The drawing under review shows one solid part. Ordinate dimensions are in mm from its lowest x, y, z. A direction names the side the tool comes from. Coordinates: 2 decimals unless noted, no trailing zeros. Write each loop counter-clockwise with the first axis right and the second up, starting at its lowest first coordinate (ties: lowest second). Pieces come first, ordered by that corner, then holes. Notation, with made-up numbers: (82.25, -2.75) - (129.25, -2.75) arc R19 ccw to (129.25, 33.25) - close; hole circle Ø10 at (5.25, -5). An arc over 180 degrees is marked (long way). Put each result on its own line as item: value. Start each with the question number.
Item 1: Machinability: for the marked faces 1 and 2, which of the approach directions +Z, -Z, +X, -X, +Y, -Y give a long, thin tool a straight path to every point of the face, cutting with its end or side? Answer none if there is none.
Item 2: Consider section B-B on z = 7.5. Give the boundary of the cut face in (x, y), then the cut area to 3 significant figures.
Item 3: Consider section A-A on x = 5.25. Give the boundary of the cut face in (y, z), then the cut area to 3 significant figures.
Item 4: To check wall thickness, follow L1, parallel to Y at x = 19, z = 1.5; L2, parallel to X at y = 37.5, z = 3.75; L3, parallel to Y at x = 11.25, z = 8. State the ranges of each line that lie inside material, in increasing order. Write a range as [from, to].
Item 5: Mouldability with a two-part tool opening along X and no side actions: class the marked faces 3, 4 and 5 as pulls with the +X half, pulls with the -X half, needs draft (parallel to the pull), parting line crosses it, or undercut.
Item 6: Consider section C-C on y = 33.5. Give the boundary of the cut face in (x, z).
Item 7: For pin 1 (10 mm diameter, centred on x = 10, y = 11, fed in from +Z), flat-tipped, find the tip position at first contact; note if it passes through.
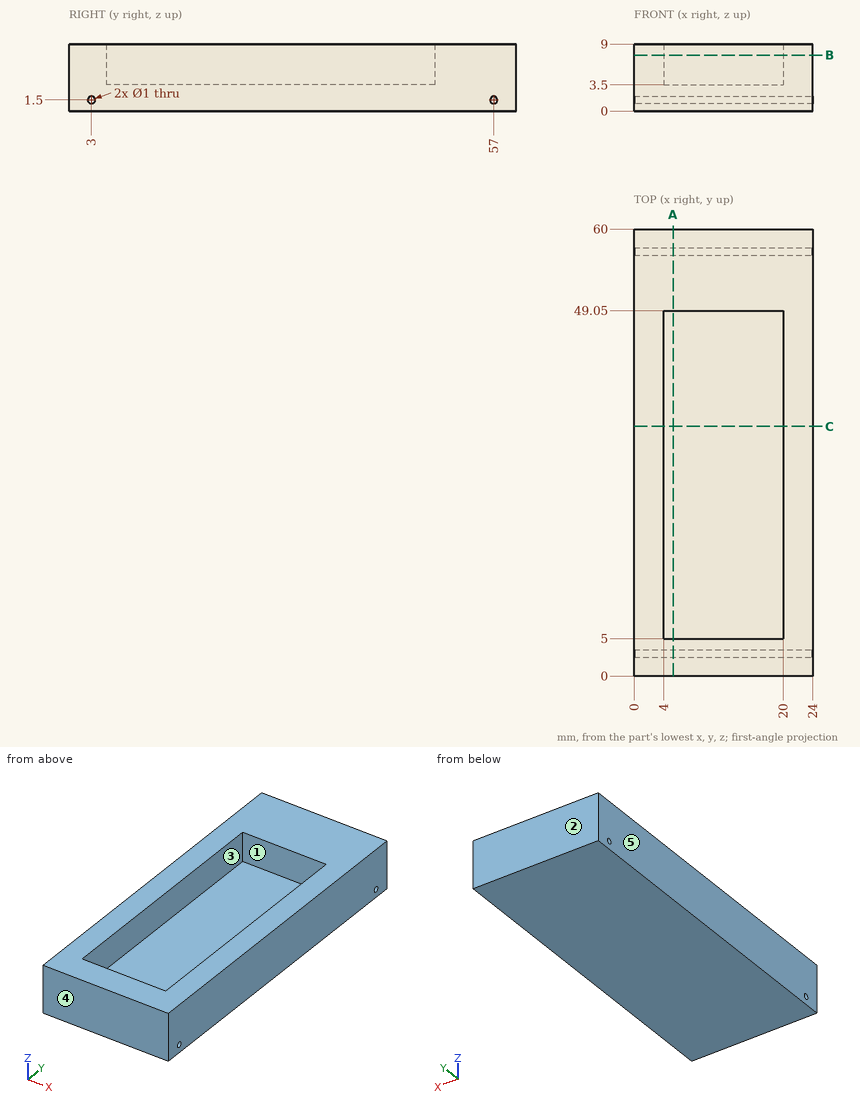
Report:
1. face 1: +Z
1. face 2: +Z, -Z, +X, -X, +Y
2. outline: (0, 0) - (24, 0) - (24, 60) - (0, 60) - close; hole (4, 5) - (20, 5) - (20, 49.05) - (4, 49.05) - close
2. area: 735 mm²
3. outline: (0, 0) - (60, 0) - (60, 9) - (49.05, 9) - (49.05, 3.5) - (5, 3.5) - (5, 9) - (0, 9) - close; hole circle Ø1 at (3, 1.5); hole circle Ø1 at (57, 1.5)
3. area: 296 mm²
4. L1: [0, 2.5], [3.5, 56.5], [57.5, 60]
4. L2: [0, 4], [20, 24]
4. L3: [0, 5], [49.05, 60]
5. face 3: undercut
5. face 4: needs draft
5. face 5: pulls with the -X half
6. outline: (0, 0) - (24, 0) - (24, 9) - (20, 9) - (20, 3.5) - (4, 3.5) - (4, 9) - (0, 9) - close
7. pin 1: z = 3.5
